from build123d import *

# Parameters (mm, degrees)
SKETCH1_W           = 64
SKETCH1_H           = 64
BOSS_EXTRUDE1_DEPTH = 8
SKETCH2_R           = 3
CUT_EXTRUDE1_DEPTH  = 28
SKETCH3_R           = 3
CUT_EXTRUDE2_DEPTH  = 28
SKETCH4_R           = 3
CUT_EXTRUDE3_DEPTH  = 28


with BuildPart() as part:
    # Sketch1 → Boss-Extrude1 (new body)
    with BuildSketch(Plane.XY.offset(300)):
        with Locations((300, 300)):
            Rectangle(SKETCH1_W, SKETCH1_H)
    extrude(amount=BOSS_EXTRUDE1_DEPTH)

    # Sketch2 → Cut-Extrude1 (cut)
    with BuildSketch(Plane.XY.offset(308)):
        with Locations((300, 300)):
            Circle(SKETCH2_R)
    extrude(amount=-CUT_EXTRUDE1_DEPTH, mode=Mode.SUBTRACT)

    # Sketch3 → Cut-Extrude2 (cut)
    with BuildSketch(Plane.XY.offset(308)):
        with Locations((300, 314)):
            Circle(SKETCH3_R)
    extrude(amount=-CUT_EXTRUDE2_DEPTH, mode=Mode.SUBTRACT)

    # Sketch4 → Cut-Extrude3 (cut)
    with BuildSketch(Plane.XY.offset(308)):
        with Locations((300, 286)):
            Circle(SKETCH4_R)
    extrude(amount=-CUT_EXTRUDE3_DEPTH, mode=Mode.SUBTRACT)


solid = part.part
Model file for the job. Use its own axes, mm. Coordinates: 2 decimals unless noted, no trailing zeros. Order: outer loops, then holes, each group sorted by start corner. A loop starts at its lowest first (then second) coordinate and runs counter-clockwise, first axis right, second up. Notation, with made-up numbers: (64, -21) -> (77, -21) arc R12 cw to (77, -8) -> close; hole circle Ø11 at (-5.75, 23.5). An arc over 180 degrees is marked (long way). Return JSON: item names as keys, results as strings. Group by question number.
Item 1: Wall check: line 1 along Y through (x, z) = (300, 303.75); line 2 along X through (y, z) = (286, 304.75); line 3 along Y through (x, z) = (302, 300.5). Give the ranges that are in metal, low to high. Write a range as [from, to].
Item 2: Pull direction X, two halves, no side cores. Call faces 1 (the flat face through (268, 300, 304)), 2 (the flat face through (300, 268, 304)), 3 (the flat face through (332, 300, 304)), 4 (the cylindrical face through (300, 289, 304)): pulls with the +X half, pulls with the -X half, needs draft (parallel to the pull), parting line crosses it, or undercut.
Item 3: Saw through at C-C on z = 305.5. Write the cut outline in (x, y), then the cut area to 3 significant figures.
Item 4: Saw through at A-A on y = 286. Write the cut outline in (x, z), then the cut area to 3 significant figures.
Item 5: Saw through at B-B on x = 300. Write the cut outline in (y, z).
Values found:
{
 "1": {"line 1": "y = [268, 283], [289, 297], [303, 311], [317, 332]", "line 2": "x = [268, 297], [303, 332]", "line 3": "y = [268, 283.76], [288.24, 297.76], [302.24, 311.76], [316.24, 332]"},
 "2": {"face 1": "pulls with the -X half", "face 2": "needs draft", "face 3": "pulls with the +X half", "face 4": "undercut"},
 "3": {"outline": "(268, 268) -> (332, 268) -> (332, 332) -> (268, 332) -> close; hole circle Ø6 at (300, 286); hole circle Ø6 at (300, 300); hole circle Ø6 at (300, 314)", "area": "4,010 mm2"},
 "4": {"outline": "(268, 300) -> (297, 300) -> (297, 308) -> (268, 308) -> close; (303, 300) -> (332, 300) -> (332, 308) -> (303, 308) -> close", "area": "464 mm2"},
 "5": {"outline": "(268, 300) -> (283, 300) -> (283, 308) -> (268, 308) -> close; (289, 300) -> (297, 300) -> (297, 308) -> (289, 308) -> close; (303, 300) -> (311, 300) -> (311, 308) -> (303, 308) -> close; (317, 300) -> (332, 300) -> (332, 308) -> (317, 308) -> close"}
}
